```python
from build123d import *

# Parameters (mm, degrees)
F1_ANGLE = 280


with BuildPart() as f1:
    # F0 (on Top) → F1 (revolve, symmetric)
    with BuildSketch(Plane.XY) as f1_sk:
        Polygon((-24.746018, 20.7264), (-34.271018, 20.7264), (-34.271018, 14.3764), (-8.871018, 14.3764), (-8.871018, 20.7264), (-18.396018, 20.7264), (-18.396018, 19.9644), (-24.746018, 19.9644), align=None)
    revolve(axis=Axis((-0.871302, 0, 0), (1, 0, 0)), revolution_arc=F1_ANGLE / 2)
    revolve(f1_sk.sketch, axis=Axis((-0.871302, 0, 0), (-1, 0, 0)), revolution_arc=F1_ANGLE / 2)


solid = f1.part
```
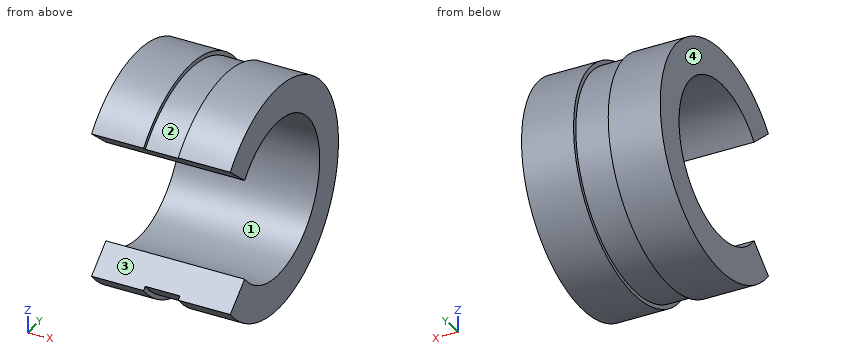
Verification items for the finished model (mm, model axes). Face numbers are marked on the shaded views. Round coordinates to 2 decimals unless told otherwise and drop trailing zeros. Write each loop counter-clockwise with the first axis right and the second up, starting at its lowest first coordinate (ties: lowest second). Pieces come first, ordered by that corner, then holes. Notation, with made-up numbers: (48, -30) -> (84, -30) arc R13 cw to (84, -13) -> close; hole circle Ø9 at (-13.75, 16). An arc over 180 degrees is marked (long way). Write each question's results on one line, items separated by ' | '.
Q1. Draft check along Z on the marked faces 1, 2, 3 and 4. Enter one of: released by +Z, released by -Z, zero draft, split by the parting line, or undercut.
Derived:
face 1: undercut | face 2: split by the parting line | face 3: undercut | face 4: zero draft
Q2. Sectioned sample at A-A, the plane y = 0. Record the boundary of the cut face in (x, z), and give its area (3 significant figures).
Derived:
outline: (-34.27, -20.73) -> (-24.75, -20.73) -> (-24.75, -19.96) -> (-18.4, -19.96) -> (-18.4, -20.73) -> (-8.87, -20.73) -> (-8.87, -14.38) -> (-34.27, -14.38) -> close; (-34.27, 14.38) -> (-8.87, 14.38) -> (-8.87, 20.73) -> (-18.4, 20.73) -> (-18.4, 19.96) -> (-24.75, 19.96) -> (-24.75, 20.73) -> (-34.27, 20.73) -> close | area: 313 mm²
Q3. Sectioned sample at B-B, the plane z = 10.5. Record the boundary of the cut face in (x, y).
Derived:
outline: (-34.27, -12.51) -> (-8.87, -12.51) -> (-8.87, -9.82) -> (-34.27, -9.82) -> close; (-34.27, 9.82) -> (-8.87, 9.82) -> (-8.87, 17.87) -> (-18.4, 17.87) -> (-18.4, 16.98) -> (-24.75, 16.98) -> (-24.75, 17.87) -> (-34.27, 17.87) -> close
Q4. Sectioned sample at C-C, the plane z = 0. Record the boundary of the cut face in (x, y).
Derived:
outline: (-34.27, 14.38) -> (-8.87, 14.38) -> (-8.87, 20.73) -> (-18.4, 20.73) -> (-18.4, 19.96) -> (-24.75, 19.96) -> (-24.75, 20.73) -> (-34.27, 20.73) -> close
Q5. Sectioned sample at D-D, the plane y = -11.5. Record the boundary of the cut face in (x, z).
Derived:
outline: (-34.27, -17.24) -> (-24.75, -17.24) -> (-24.75, -16.32) -> (-18.4, -16.32) -> (-18.4, -17.24) -> (-8.87, -17.24) -> (-8.87, -9.65) -> (-34.27, -9.65) -> close; (-34.27, 9.65) -> (-8.87, 9.65) -> (-8.87, 17.24) -> (-18.4, 17.24) -> (-18.4, 16.32) -> (-24.75, 16.32) -> (-24.75, 17.24) -> (-34.27, 17.24) -> close
Q6. Thickness scan on probe 1 along Z at (x, y) = (-22, 0); probe 2 along Z at (x, y) = (-28.5, 0); probe 3 along Y at (x, z) = (-18.25, 0). Record the ranges inside material, lowest first.
Derived:
probe 1: z = -19.96 to -14.38, 14.38 to 19.96 | probe 2: z = -20.73 to -14.38, 14.38 to 20.73 | probe 3: y = 14.38 to 20.73
Q7. Go/stop test with flat-tipped pins: pin 1 Ø1.5 at (x, z) = (-22, 16) entering from +Y; pin 2 Ø1.5 at (x, z) = (-14, -11.5) entering from +Y; pin 3 Ø1.5 at (x, y) = (-17.5, -2) entering from -Z; pin 4 Ø8 at (y, z) = (0, -8.5) entering from +X. Record where each tip stops, or that it passes through.
Derived:
pin 1: stops at y = 12.88 | pin 2: stops at y = 17.72 | pin 3: stops at z = -20.69 | pin 4: passes through
